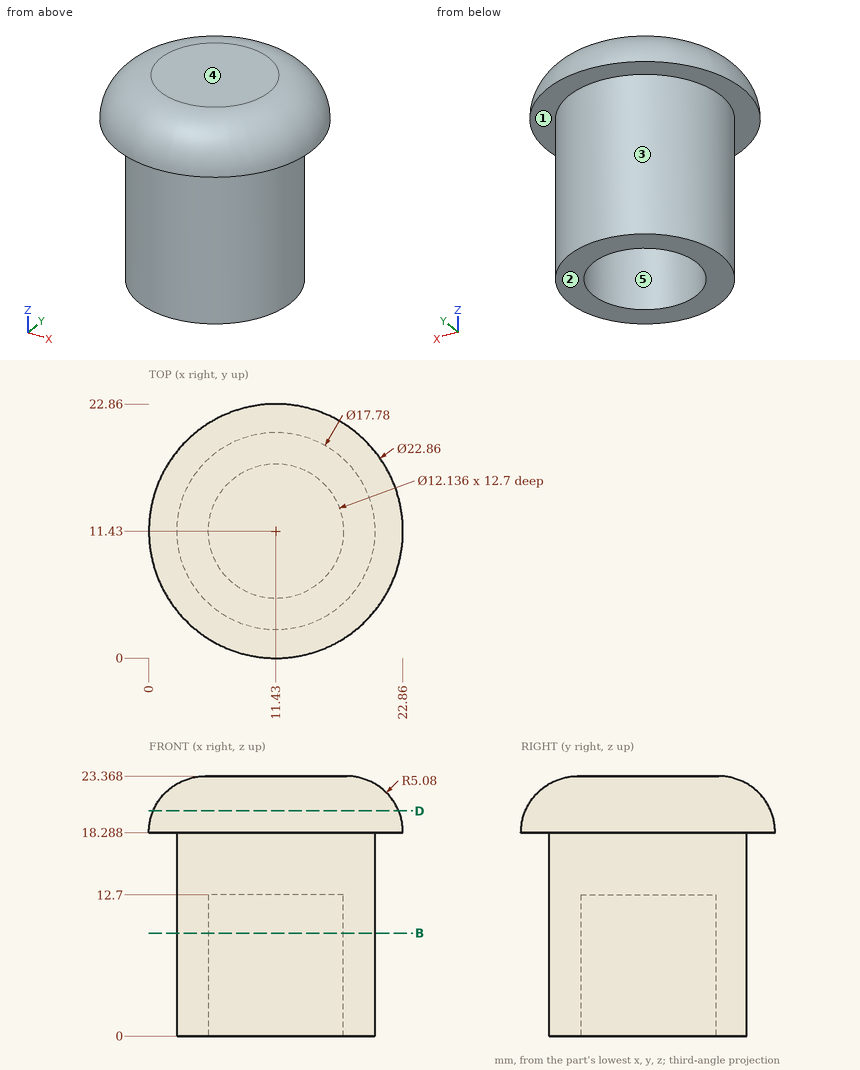
Input: dimensioned drawing with shaded views. Units: mm. Origin: part minimum x, y, z. A direction names the side the tool comes from. Coordinates: 2 decimals unless noted, no trailing zeros. Order: outer loops, then holes, each group sorted by start corner. A loop starts at its lowest first (then second) coordinate and runs counter-clockwise, first axis right, second up. Notation, with made-up numbers: (87, 75) - (130, 75) arc R27 cw to (130, 114) - close; hole circle Ø10 at (35, 43). An arc over 180 degrees is marked (long way). Return JSON: item names as keys, results as strings. Group by question number.
1. Material intervals for line 1 along Y through (x, z) = (11.43, 9.75); line 2 along Y through (x, z) = (6, 4.75), sorted ascending. Write a range as [from, to].
2. Cut plane B-B (z = 9.25). Output: boundary loops of the cut face in (x, y).
3. Set-up query: the marked faces 1 and 2. Return all of +Z, -Z, +X, -X, +Y, -Y with unobstructed straight access to the full face (end or side cutting, diameter ignored); none if empty.
4. Pin query (flat end, axial travel): pin 1 (12 mm diameter, centred on x = 8.5, z = 9, fed in from -Y); pin 2 (3 mm diameter, centred on x = 16.5, y = 20, fed in from +Z); pin 3 (12 mm diameter, centred on x = 11, z = 6, fed in from +Y). Return the tip coordinate at first contact, or that it passes through.
5. Pull-direction query (Y, two-part tool) for the marked faces 3, 4 and 5; classes: pulls with the +Y half, pulls with the -Y half, needs draft (parallel to the pull), parting line crosses it, or undercut.
6. Cut plane D-D (z = 20.25). Output: boundary loops of the cut face in (x, y).
Resolved:
{
 "1": {"line 1": "y = [2.54, 5.36], [17.5, 20.32]", "line 2": "y = [4.39, 8.72], [14.14, 18.47]"},
 "2": {"outline": "circle Ø17.78 at (11.43, 11.43); hole circle Ø12.14 at (11.43, 11.43)"},
 "3": {"face 1": "-Z", "face 2": "-Z, +X, -X, +Y, -Y"},
 "4": {"pin 1": "stops at y = 2.54", "pin 2": "stops at z = 22.91", "pin 3": "stops at y = 20.32"},
 "5": {"face 3": "parting line crosses it", "face 4": "needs draft", "face 5": "undercut"},
 "6": {"outline": "circle Ø22.07 at (11.43, 11.43)"}
}
